Here's the drawing with two shaded views (mm, measured from the low corner). I have some questions. Coordinates: 2 decimals unless noted, no trailing zeros. Loops run counter-clockwise (first coordinate to the right, second up) from the corner with the lowest first, then second, coordinate; pieces in that order, holes last.
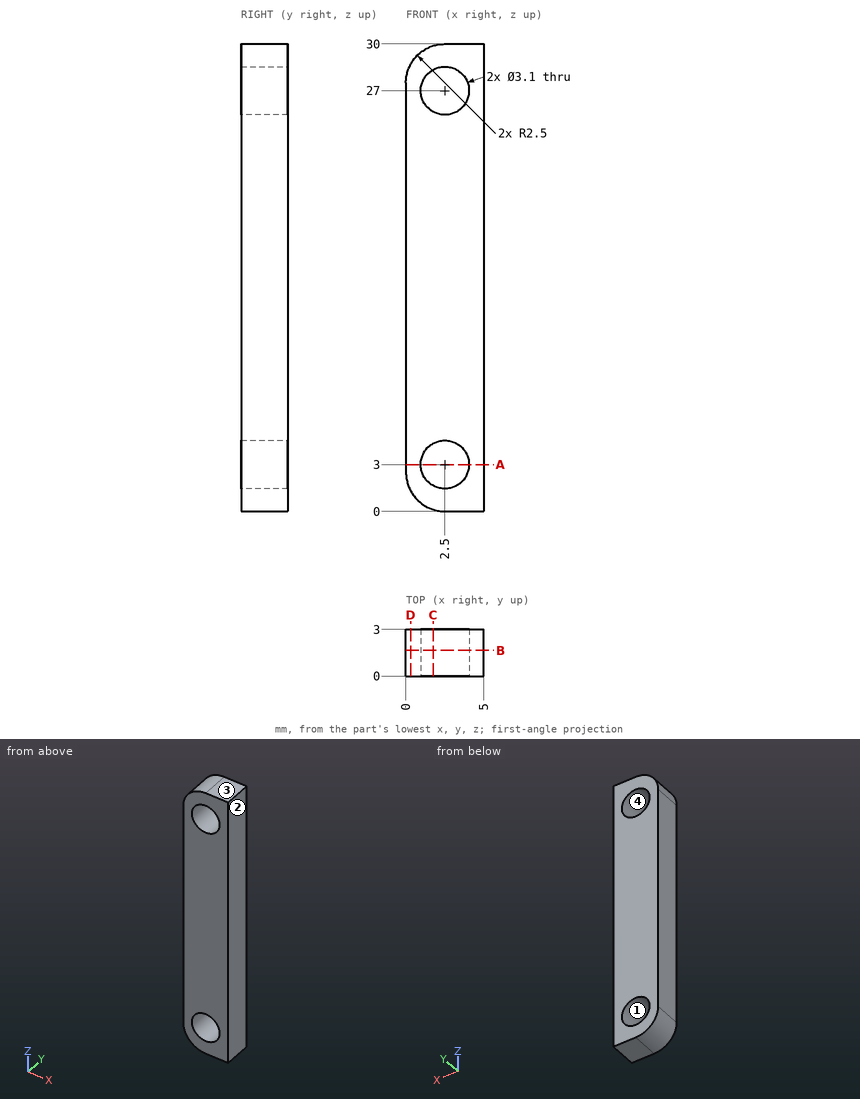
(1) I want a section at C-C on x = 1.75. Write out the boundary of the cut face in (y, z).
Check values:
outline: (0, 0.12) - (3, 0.12) - (3, 1.64) - (0, 1.64) - close; (0, 4.36) - (3, 4.36) - (3, 25.64) - (0, 25.64) - close; (0, 28.36) - (3, 28.36) - (3, 29.88) - (0, 29.88) - close
(2) I want a section at D-D on x = 0.3. Write out the boundary of the cut face in (y, z), then the cut area to 3 significant figures.
Check values:
outline: (0, 1.31) - (3, 1.31) - (3, 28.69) - (0, 28.69) - close
area: 82.1 mm2
(3) I want a section at A-A on z = 3. Write out the boundary of the cut face in (x, y), then the cut area to 3 significant figures.
Check values:
outline: (0, 0) - (0.95, 0) - (0.95, 3) - (0, 3) - close; (4.05, 0) - (5, 0) - (5, 3) - (4.05, 3) - close
area: 5.70 mm2
(4) If I drill on probe 1 along X at (y, z) = (0.65, 27); probe 2 along Z at (x, y) = (3.1, 0.4); probe 3 along Z at (x, y) = (1.45, 0.55), over which ranges is the centre line in solid material (lowest first)?
Check values:
probe 1: x = 0 to 0.95, 4.05 to 5
probe 2: z = 0 to 1.57, 4.43 to 25.57, 28.43 to 30
probe 3: z = 0.23 to 1.86, 4.14 to 25.86, 28.14 to 29.77
(5) If we mould it in two halves opening along X, with no side actions, what happens to the marked faces 1, 2, 3 and 4? For each: released by +X, released by -X, zero draft, split by the parting line, or undercut.
Check values:
face 1: undercut
face 2: released by +X
face 3: zero draft
face 4: undercut
(6) I want a section at B-B on y = 1.65. Write out the boundary of the cut face in (x, z), then the cut area to 3 significant figures.
Check values:
outline: (0, 2.5) arc R2.5 ccw to (2.5, 0) - (5, 0) - (5, 30) - (2.5, 30) arc R2.5 ccw to (0, 27.5) - close; hole circle Ø3.1 at (2.5, 3); hole circle Ø3.1 at (2.5, 27)
area: 132 mm2
